Input: part model. Units: mm. Frame: model coordinates. A direction names the side the tool comes from. Coordinates: 2 decimals unless noted, no trailing zeros. Loops run counter-clockwise (first coordinate to the right, second up) from the corner with the lowest first, then second, coordinate; pieces in that order, holes last. Notation, with made-up numbers: (4, 37.5) -> (22, 37.5) arc R20 ccw to (22, 76.5) -> close; hole circle Ø6 at (50, 69). An arc over 180 degrees is marked (long way). Put each result on its own line as item: value. Start each with the question number.
1) Cut plane C-C (z = 6). Return the cut outline in (x, y).
2) Contact query for flat-ended pins moving along their axis: P1, Ø4, axis at x = 18.5, z = 4.5, coming from the +Y side; P2, Ø1.1, axis at y = 16.5, z = 5, coming from the +X side; P3, Ø4, axis at x = 74, y = 5, coming from the +Z side; P4, Ø5, axis at x = 67.5, y = 11.5, coming from the +Z side. Output: stop coordinate, or through.
3) Cut plane B-B (y = 13.25). Return the cut outline in (x, z).
4) Cut plane D-D (x = 54.5). Return the cut outline in (y, z).
5) Cut plane A-A (x = 74). Return the cut outline in (y, z).
6) Set-up query: faces 1 (the flat face through (64, 16, 6)), 2 (the flat face through (38, 18, 5)), 3 (the flat face through (39, 20, 1)). Return all of +Z, -Z, +X, -X, +Y, -Y with unobstructed straight access to the full face (end or side cutting, diameter ignored); none if empty.
7) Material intervals for L1, parallel to X at y = 5, z = 1.45; L2, parallel to Z at x = 43, y = 16; L3, parallel to Y at x = 6, z = 1.75, sorted ascending.
8) Pull-direction query (Y, two-part tool) for faces 4 (the flat face through (39, 0, 1)), 5 (the cylindrical face through (51.182, 17.4, 7.284)), 6 (the cylindrical face through (76.196, 4.512, 1.232)), 7 (the flat face through (80, 10, 1)); classes: pulls with the +Y half, pulls with the -Y half, needs draft (parallel to the pull), parting line crosses it, or undercut.
from build123d import *

# Parameters (mm, degrees)
BOX_W             = 80
BOX_H             = 20
BOX_DEPTH         = 2.5
CYLINDER_R        = 4
CYLINDER_DEPTH    = 38
CYLINDER001_R     = 1.9
CYLINDER001_DEPTH = 30
CYLINDER002_R     = 2.25
CYLINDER002_DEPTH = 2.5
CYLINDER003_R     = 2.25
CYLINDER003_DEPTH = 2.5


with BuildPart() as part:
    # Box → Box (join)
    with BuildSketch(Plane.XY):
        with Locations((40, 10)):
            Rectangle(BOX_W, BOX_H)
    extrude(amount=BOX_DEPTH)

    # Cylinder → Cylinder (join)
    with BuildSketch(Plane(origin=(38, 16, 6), x_dir=(0, -1, 0), z_dir=(-1, 0, 0))):
        Circle(CYLINDER_R)
    extrude(amount=CYLINDER_DEPTH)

    # Cylinder001 → Cylinder001 (join)
    with BuildSketch(Plane(origin=(64, 16, 6), x_dir=(0, -1, 0), z_dir=(-1, 0, 0))):
        Circle(CYLINDER001_R)
    extrude(amount=CYLINDER001_DEPTH)

    # Cylinder002 → Cylinder002 (cut)
    with BuildSketch(Plane(origin=(74, 5, 0), x_dir=(0, 1, 0), z_dir=(0, 0, 1))):
        Circle(CYLINDER002_R)
    extrude(amount=CYLINDER002_DEPTH, mode=Mode.SUBTRACT)

    # Cylinder003 → Cylinder003 (cut)
    with BuildSketch(Plane(origin=(6, 5, 0), x_dir=(0, 1, 0), z_dir=(0, 0, 1))):
        Circle(CYLINDER003_R)
    extrude(amount=CYLINDER003_DEPTH, mode=Mode.SUBTRACT)


solid = part.part
Results found:
1. outline: (0, 12) -> (38, 12) -> (38, 14.1) -> (64, 14.1) -> (64, 17.9) -> (38, 17.9) -> (38, 20) -> (0, 20) -> close
2. P1: stops at y = 20
2. P2: stops at x = 64
2. P3: passes through
2. P4: stops at z = 2.5
3. outline: (0, 0) -> (80, 0) -> (80, 2.5) -> (0, 2.5) -> close; (0, 3.1) -> (38, 3.1) -> (38, 8.9) -> (0, 8.9) -> close
4. outline: (0, 0) -> (20, 0) -> (20, 2.5) -> (0, 2.5) -> close; circle Ø3.8 at (16, 6)
5. outline: (0, 0) -> (2.75, 0) -> (2.75, 2.5) -> (0, 2.5) -> close; (7.25, 0) -> (20, 0) -> (20, 2.5) -> (7.25, 2.5) -> close
6. face 1: +Z, +X, +Y, -Y
6. face 2: +X
6. face 3: +Z, -Z, +X, -X, +Y
7. L1: x = 0 to 3.75, 8.25 to 71.75, 76.25 to 80
7. L2: z = 0 to 2.5, 4.1 to 7.9
7. L3: y = 0 to 2.75, 7.25 to 20
8. face 4: pulls with the -Y half
8. face 5: parting line crosses it
8. face 6: undercut
8. face 7: needs draft
